Part model, mm, in its own coordinate system. A direction names the side the tool comes from. Round coordinates to 2 decimals unless told otherwise and drop trailing zeros. Write each loop counter-clockwise with the first axis right and the second up, starting at its lowest first coordinate (ties: lowest second). Pieces come first, ordered by that corner, then holes. Notation, with made-up numbers: M -18.5,28.5 L -14.5,28.5 A12 cw -14.5,40.5 Z; hole C -23.5,75 d11. An arc over 180 degrees is marked long. Answer as a JSON object with one key per item and string values. Group by question number.
1. Which spindle directions (+Z, -Z, +X, -X, +Y, -Y) get a long thin tool onto all of the face, cutting with end or side? Do faces 5 (the face through (-6, -85, 101.6)), 6 (the face through (-12, -88, 111.125)), 7 (the face through (-3, -72.47, -120)). Say none if no direction does.
2. Two-plate mould, pull along Z, no slides. Class faces 1 (the face through (25, -128, 342.9)), 2 (the face through (-6, -85, -101.6)), 3 (the face through (-3, -72.47, 121)), 4 (the face through (-5, -85, -139.7)): +Z half, -Z half, draft (parallel to the pull), parting line (faces both ways), or undercut.
3. Band-saw the part on A-A, the plane z = -147.5. Write the cut outline in (x, y) (1 decimal), plus the area to 3 significant figures.
4. Drill centre lines: line 1 (X direction, y = -139, z = -23.5); line 2 (X direction, y = -74, z = 243); line 3 (Y direction, x = 33, z = -150). Where is each one in solid material? Low to high. Write a range as from..to.
5. Drop flat-ended pins along their axis: pin 1 (7 mm diameter, centred on x = -4, z = 115.5, fed in from +Y); pin 2 (20.5 mm diameter, centred on x = -2, y = -85, fed in from +Z); pin 3 (12 mm diameter, centred on x = 31, z = -131.5, fed in from -Y); pin 4 (10 mm diameter, centred on y = -194, z = -246.5, fed in from -X). Give the stop position or say it passes through.
6. Band-saw the part on B-B, the plane y = -54.5. Write the cut outline in (x, z), plus the area to 3 significant figures.
from build123d import *

# Parameters (mm, degrees)
EXTRUDE_THIN1_DEPTH = 342.9
BOSS_EXTRUDE1_START = -203.2
BOSS_EXTRUDE1_DEPTH = 279.4
CUT_EXTRUDE1_START  = -38.1
CUT_EXTRUDE1_DEPTH  = 203.2
CUT_EXTRUDE2_START  = -9.525
SKETCH4_R           = 3.048
CUT_EXTRUDE2_DEPTH  = 19.05
CUT_EXTRUDE3_START  = -28.575
SKETCH5_R           = 3.048
CUT_EXTRUDE3_DEPTH  = 19.05


with BuildPart() as part:
    # Sketch1 → Extrude-Thin1 (new, symmetric)
    with BuildSketch(Plane.XY):
        with BuildLine():
            ThreePointArc((0, 0), (28.7854342, -135.80582632), (101.6, -254))
            Line((101.6, -254), (98.031425453, -257.153836069))
            ThreePointArc((98.031425453, -257.153836069), (24.36356396, -137.574574416), (-4.759199547, -0.177273569))
            Line((-4.759199547, -0.177273569), (0, 0))
        make_face()
    extrude(amount=EXTRUDE_THIN1_DEPTH, both=True)

    # Sketch2 → Boss-Extrude1 (add)
    with BuildSketch(Plane.XY.offset(342.9).offset(BOSS_EXTRUDE1_START)):
        with BuildLine():
            Line((-9.288950239, -72.469656114), (4.395363676, -72.469656114))
            ThreePointArc((4.395363676, -72.469656114), (7.38925865, -85.220570454), (10.787766498, -97.869656114))
            Line((10.787766498, -97.869656114), (-9.288950239, -97.869656114))
            ThreePointArc((-9.288950239, -97.869656114), (-21.988950239, -85.169656114), (-9.288950239, -72.469656114))
        make_face()
    extrude(amount=-BOSS_EXTRUDE1_DEPTH)

    # Sketch3 → Cut-Extrude1 (cut)
    with BuildSketch(Plane.XY.offset(139.7).offset(CUT_EXTRUDE1_START)):
        with BuildLine():
            Line((-9.288950239, -97.869656114), (10.787766498, -97.869656114))
            ThreePointArc((10.787766498, -97.869656114), (7.38925865, -85.220570454), (4.395363676, -72.469656114))
            Line((4.395363676, -72.469656114), (-9.288950239, -72.469656114))
            ThreePointArc((-9.288950239, -72.469656114), (-21.988950239, -85.169656114), (-9.288950239, -97.869656114))
        make_face()
    extrude(amount=-CUT_EXTRUDE1_DEPTH, mode=Mode.SUBTRACT)

    # Sketch4 → Cut-Extrude2 (cut)
    with BuildSketch(Plane.XY.offset(-101.6).offset(CUT_EXTRUDE2_START)):
        with BuildLine():
            ThreePointArc((-9.288950239, -97.869656114), (-0.308694117, -94.149912235), (3.411049761, -85.169656114))
            ThreePointArc((3.411049761, -85.169656114), (-0.308694117, -76.189399993), (-9.288950239, -72.469656114))
            ThreePointArc((-9.288950239, -72.469656114), (-21.988950239, -85.169656114), (-9.288950239, -97.869656114))
        make_face()
        with Locations((-9.288950239, -85.169656114)):
            Circle(SKETCH4_R, mode=Mode.SUBTRACT)
    extrude(amount=-CUT_EXTRUDE2_DEPTH, mode=Mode.SUBTRACT)

    # Sketch5 → Cut-Extrude3 (cut)
    with BuildSketch(Plane(origin=(0, 0, 101.6), x_dir=(-1, 0, 0), z_dir=(0, 0, -1)).offset(CUT_EXTRUDE3_START)):
        with BuildLine():
            ThreePointArc((9.288950239, -97.869656114), (18.26920636, -94.149912235), (21.988950239, -85.169656114))
            ThreePointArc((21.988950239, -85.169656114), (18.26920636, -76.189399993), (9.288950239, -72.469656114))
            ThreePointArc((9.288950239, -72.469656114), (-3.411049761, -85.169656114), (9.288950239, -97.869656114))
        make_face()
        with Locations(Location((9.288950239, -85.169656114, 0), (0, 0, 180))):
            Circle(SKETCH5_R, mode=Mode.SUBTRACT)
    extrude(amount=CUT_EXTRUDE3_DEPTH, mode=Mode.SUBTRACT)


solid = part.part
Worked answers:
{
 "1": {"face 5": "-X, -Y", "face 6": "none", "face 7": "+Z, -Z, -X"},
 "2": {"face 1": "+Z half", "face 2": "undercut", "face 3": "draft", "face 4": "-Z half"},
 "3": {"outline": "M -4.8,-0.2 A411.2 ccw 98,-257.2 L 101.6,-254 A406.4 cw 0,0 Z", "area": "1,340 mm^2"},
 "4": {"line 1": "x = 24.94..30.08", "line 2": "x = 4.73..9.61", "line 3": "y = -157.61..-145.94"},
 "5": {"pin 1": "stops at y = -0.02", "pin 2": "stops at z = 342.9", "pin 3": "stops at y = -166", "pin 4": "stops at x = 49.21"},
 "6": {"outline": "M 0.89,-342.9 L 5.73,-342.9 L 5.73,342.9 L 0.89,342.9 Z", "area": "3,310 mm^2"}
}
